```python
from build123d import *

# Parameters (mm, degrees)
SKETCH1_W                                            = 59.1
SKETCH1_H                                            = 59.1
BOSS_EXTRUDE1_DEPTH                                  = 59.1
CUT_EXTRUDE1_DEPTH                                   = 94.96477218
CUT_EXTRUDE1_DEPTH_BACK                              = 3.5
SKETCH2_W                                            = 96.91536242
SKETCH2_H                                            = 99.114771323
FILLET1_R                                            = 7.5
SHELL1_T                                             = -2.5
CSK_SLOT_FOR_M2_COUNTERSUNK_FLAT_HEAD_SC_D           = 2.4
CSK_SLOT_FOR_M2_COUNTERSUNK_FLAT_HEAD_SC_CSINK_D     = 4.4
CSK_SLOT_FOR_M2_COUNTERSUNK_FLAT_HEAD_SC_CSINK_ANGLE = 90
CUT_EXTRUDE2_DEPTH                                   = 45.76614234


with BuildPart() as part:
    # Sketch1 → Boss-Extrude1 (new body)
    with BuildSketch(Plane.XY):
        Rectangle(SKETCH1_W, SKETCH1_H)
    extrude(amount=BOSS_EXTRUDE1_DEPTH)

    # Sketch2 → Cut-Extrude1 (cut, two sides: drawn at the far end of the back side and taken through both)
    with BuildSketch(Plane(origin=(30.720954492, 30.720954492, 39.55), x_dir=(0.2588190451025209, -0.9659258262890682, 0), z_dir=(0, 0, -1)).offset(-CUT_EXTRUDE1_DEPTH_BACK)):
        with Locations((21.755390695, 38.565126259)):
            Rectangle(SKETCH2_W, SKETCH2_H)
    extrude(amount=CUT_EXTRUDE1_DEPTH + CUT_EXTRUDE1_DEPTH_BACK, mode=Mode.SUBTRACT)

    # Fillet1
    fillet1_edges = [part.edges().sort_by_distance(p)[0] for p in [
        (29.55, 0, 59.1),
        (0, 29.55, 59.1),
        (-29.55, 0, 59.1),
        (0, -29.55, 59.1),
        (-29.55, 29.55, 51.075),
        (29.55, 29.55, 51.075),
        (29.55, -29.55, 51.075),
        (-29.55, -29.55, 51.075),
    ]]
    fillet(fillet1_edges, radius=FILLET1_R)

    # Shell1
    shell1_openings = [part.faces().sort_by_distance(p)[0] for p in [
        (0, 0, 43.05),
    ]]
    offset(amount=SHELL1_T, openings=shell1_openings, kind=Kind.INTERSECTION)

    # CSK SLOT for M2 Countersunk Flat Head Screw1 (through all)
    with Locations(Plane.XY.offset(59.1)):
        with Locations((16, 16), (19.892963711, -96.835353), (-16, -16)):
            CounterSinkHole(CSK_SLOT_FOR_M2_COUNTERSUNK_FLAT_HEAD_SC_D / 2, CSK_SLOT_FOR_M2_COUNTERSUNK_FLAT_HEAD_SC_CSINK_D / 2, counter_sink_angle=CSK_SLOT_FOR_M2_COUNTERSUNK_FLAT_HEAD_SC_CSINK_ANGLE)

    # Sketch20 → Cut-Extrude2 (cut, through all)
    with BuildSketch(Plane.XY.offset(59.1)):
        Polygon((-1.825, -3.160992724), (1.825, -3.160992724), (3.65, 0), (1.825, 3.160992724), (-1.825, 3.160992724), (-3.65, 0), align=None)
    extrude(amount=-CUT_EXTRUDE2_DEPTH, mode=Mode.SUBTRACT)


solid = part.part
```
The listing builds one solid part. Answer for the finished solid, in the listing's coordinates (mm). A direction names the side the tool comes from. Coordinates: 2 decimals unless noted, no trailing zeros. Loops run counter-clockwise (first coordinate to the right, second up) from the corner with the lowest first, then second, coordinate; pieces in that order, holes last. Notation, with made-up numbers: (40, 49) -> (71, 49) arc R29 ccw to (71, 86) -> close; hole circle Ø5 at (-37.5, -11.5). An arc over 180 degrees is marked (long way). Use one line per item in the form item = value. Start each with the question number.
Item 1: The part is cut by section D-D on x = 11.5. Determine the outline of the cut face in (y, z).
Item 2: The part is cut by section B-B on y = 16. Determine the outline of the cut face in (x, z), then the cut area to 3 significant figures.
Item 3: A tool of negligible diameter and unlimited length cuts with its end or side. For faces 5 (the face through (-27.411, -27.295, 47.385)), 6 (the face through (0.31, -25.55, 55.17)), 7 (the face through (0, 3.161, 58)), from which of +Z, -Z, +X, -X, +Y, -Y can it reach the whole face along a straight path? Write none if from no direction.
Item 4: Consider L1, parallel to X at y = 20, z = 52; L2, parallel to X at y = 10.5, z = 44.5; L3, parallel to Z at x = 20.5, y = -5.5. Determine where each line is inside the solid, lowest interval first. Write a range as [from, to].
Item 5: The mould has two halves that part along X. Classify faces 1 (the face through (2.725, -1.603, 57.868)), 2 (the face through (29.55, 0, 47)), 3 (the face through (-16.554, -17.065, 57.34)), 4 (the face through (0.309, 27.411, 56.845)): released by +X, released by -X, zero draft, split by the parting line, or undercut.
Item 6: Flat-ended cylindrical pins translate along their axes: pin 1 Ø2 at (x, z) = (10, 54) entering from +Y; pin 2 Ø0.8 at (x, z) = (0, 57.5) entering from +Y; pin 3 Ø1.2 at (x, z) = (0.5, 58.5) entering from -Y. Find the tip coordinate at first contact, or state that the pin passes through.
Item 7: The part is cut by section A-A on z = 50.25. Determine the outline of the cut face in (x, y).
Item 8: The part is cut by section C-C on x = -0.5. Determine the outline of the cut face in (y, z).
Answer key:
q1.outline = (-29.55, 43.05) -> (-27.05, 43.05) -> (-27.05, 51.6) arc R5 cw to (-22.05, 56.6) -> (22.05, 56.6) arc R5 cw to (27.05, 51.6) -> (27.05, 43.05) -> (29.55, 43.05) -> (29.55, 51.6) arc R7.5 ccw to (22.05, 59.1) -> (-22.05, 59.1) arc R7.5 ccw to (-29.55, 51.6) -> close
q2.outline = (-29.55, 43.05) -> (-27.05, 43.05) -> (-27.05, 51.6) arc R5 cw to (-22.05, 56.6) -> (14.8, 56.6) -> (14.8, 58.1) -> (13.8, 59.1) -> (-22.05, 59.1) arc R7.5 ccw to (-29.55, 51.6) -> close; (17.2, 56.6) -> (22.05, 56.6) arc R5 cw to (27.05, 51.6) -> (27.05, 43.05) -> (29.55, 43.05) -> (29.55, 51.6) arc R7.5 ccw to (22.05, 59.1) -> (18.2, 59.1) -> (17.2, 58.1) -> close
q2.area = 195 mm2
q3.face_5 = +Z, -Z, -X, -Y
q3.face_6 = -Z
q3.face_7 = +Z, -Z
q4.L1 = [-29.54, -27.03], [27.03, 29.54]
q4.L2 = [-29.55, -27.05], [27.05, 29.55]
q4.L3 = [56.6, 59.1]
q5.face_1 = undercut
q5.face_2 = released by +X
q5.face_3 = undercut
q5.face_4 = zero draft
q6.pin_1 = 29.42
q6.pin_2 = 27.15
q6.pin_3 = -26.12
q7.outline = (-29.55, -22.05) arc R7.5 ccw to (-22.05, -29.55) -> (22.05, -29.55) arc R7.5 ccw to (29.55, -22.05) -> (29.55, 22.05) arc R7.5 ccw to (22.05, 29.55) -> (-22.05, 29.55) arc R7.5 ccw to (-29.55, 22.05) -> close; hole (-27.05, -22.05) arc R5 ccw to (-22.05, -27.05) -> (22.05, -27.05) arc R5 ccw to (27.05, -22.05) -> (27.05, 22.05) arc R5 ccw to (22.05, 27.05) -> (-22.05, 27.05) arc R5 ccw to (-27.05, 22.05) -> close
q8.outline = (-29.55, 43.05) -> (-27.05, 43.05) -> (-27.05, 51.6) arc R5 cw to (-22.05, 56.6) -> (-3.16, 56.6) -> (-3.16, 59.1) -> (-22.05, 59.1) arc R7.5 ccw to (-29.55, 51.6) -> close; (3.16, 56.6) -> (22.05, 56.6) arc R5 cw to (27.05, 51.6) -> (27.05, 43.05) -> (29.55, 43.05) -> (29.55, 51.6) arc R7.5 ccw to (22.05, 59.1) -> (3.16, 59.1) -> close
